Design review of the part built by this model. Coordinates are the model's own, in mm. Face numbers are marked on the shaded views. A direction names the side the tool comes from. Give positions to 0.01 mm unless a question says otherwise; leave off trailing zeros. Write each loop counter-clockwise with the first axis right and the second up, starting at its lowest first coordinate (ties: lowest second). Pieces come first, ordered by that corner, then holes. Notation, with made-up numbers: (77.5, 20.5) -> (124.5, 20.5) arc R27 cw to (124.5, 37.5) -> close; hole circle Ø2 at (37.25, -30.75). An arc over 180 degrees is marked (long way). Return JSON: item names as keys, results as strings. Group by question number.
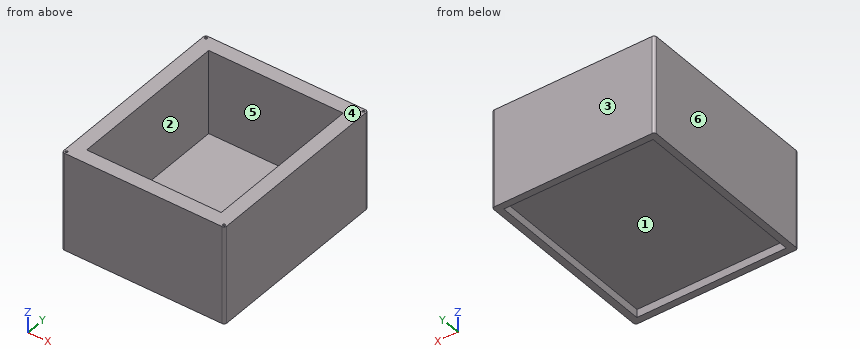
from build123d import *

# Parameters (mm, degrees)
F0_W     = 61.468
F0_H     = 71.628
F0_W_2   = 50.8
F0_H_2   = 60.96
F1_DEPTH = 18.542
F2_W     = 50.8
F2_H     = 60.96
F3_DEPTH = 5.334
F4_R     = 0.9906
F5_T     = -2.54
F6_R     = 0.4445
F7_DEPTH = 3.3782


with BuildPart() as f1:
    # F0 (on Top) → F1 (new body, symmetric)
    with BuildSketch(Plane.XY):
        Rectangle(F0_W, F0_H)
        Rectangle(F0_W_2, F0_H_2, mode=Mode.SUBTRACT)
    extrude(amount=F1_DEPTH, both=True)

    # F2 (on face) → F3 (join)
    with BuildSketch(Plane(origin=(0, 0, -18.542), x_dir=(1, 0, 0), z_dir=(0, 0, -1))):
        Rectangle(F2_W, F2_H)
    extrude(amount=-F3_DEPTH)

    # F4
    f4_edges = [f1.edges().sort_by_distance(p)[0] for p in [
        (-30.734, 35.814, 0),
        (30.734, 35.814, 0),
        (30.734, -35.814, 0),
        (-30.734, -35.814, 0),
    ]]
    fillet(f4_edges, radius=F4_R)

    # F5
    f5_openings = [f1.faces().sort_by_distance(p)[0] for p in [
        (0, 0, -18.542),
    ]]
    offset(amount=F5_T, openings=f5_openings, kind=Kind.INTERSECTION)

    # F6 (on face) → F7 (cut)
    with BuildSketch(Plane.XY.offset(18.542)):
        with Locations((-29.7434, 34.8234)):
            Circle(F6_R)
        with Locations((29.7434, 34.8234)):
            Circle(F6_R)
        with Locations((29.7434, -34.8234)):
            Circle(F6_R)
        with Locations((-29.7434, -34.8234)):
            Circle(F6_R)
    extrude(amount=-F7_DEPTH, mode=Mode.SUBTRACT)


solid = f1.part
Q1. Mouldability with a two-part tool opening along X and no side actions: class the marked faces 4, 5 and 6 as +X half, -X half, draft (parallel to the pull), parting line (faces both ways), or undercut.
Q2. Take a section at A-A, the plane z = 0. Give the boundary of the cut face in (x, y), plus the area to 3 significant figures.
Q3. Insertion check: pin 1 (12 mm diameter, centred on x = 15, y = -25.5, fed in from -Z); pin 2 (6 mm diameter, centred on x = -1, y = 16.5, fed in from +Z). Each pin has a flat end and moves straight along its axis. Give the tip position at first contact, or say it passes through.
Q4. Take a section at C-C, the plane y = 15. Give the boundary of the cut face in (x, z).
Q5. Tool access review of the marked faces 1, 2 and 3: name each direction out of +Z, -Z, +X, -X, +Y, -Y from which nothing blocks a thin tool from reaching the whole face with its end or side.
Q6. Take a section at B-B, the plane x = 19.5. Give the boundary of the cut face in (y, z).
Q7. For L1, parallel to X at y = -28, z = 5.5; L2, parallel to Y at x = 26, z = -4; L3, parallel to Y at x = 19, z = 15, list the stretches that pass through material, from the lowest coordinate up. Write a range as from..to.
Final values:
{
 "1": {"face 4": "draft", "face 5": "undercut", "face 6": "-X half"},
 "2": {"outline": "(-30.73, -34.82) arc R0.99 ccw to (-29.74, -35.81) -> (29.74, -35.81) arc R0.99 ccw to (30.73, -34.82) -> (30.73, 34.82) arc R0.99 ccw to (29.74, 35.81) -> (-29.74, 35.81) arc R0.99 ccw to (-30.73, 34.82) -> close; (-27.94, -33.02) -> (27.94, -33.02) -> (27.94, 33.02) -> (-27.94, 33.02) -> close; hole (-28.19, -33.27) -> (28.19, -33.27) -> (28.19, 33.27) -> (-28.19, 33.27) -> close; hole (-25.4, -30.48) -> (25.4, -30.48) -> (25.4, 30.48) -> (-25.4, 30.48) -> close", "area": "1,240 mm²"},
 "3": {"pin 1": "stops at z = -15.75", "pin 2": "stops at z = -13.21"},
 "4": {"outline": "(-30.73, -18.54) -> (-28.19, -18.54) -> (-28.19, 16) -> (-27.94, 16) -> (-27.94, -15.75) -> (27.94, -15.75) -> (27.94, 16) -> (28.19, 16) -> (28.19, -18.54) -> (30.73, -18.54) -> (30.73, 18.54) -> (25.4, 18.54) -> (25.4, -13.21) -> (-25.4, -13.21) -> (-25.4, 18.54) -> (-30.73, 18.54) -> close"},
 "5": {"face 1": "-Z", "face 2": "+Z", "face 3": "+Z, -Z, +X, -X, +Y"},
 "6": {"outline": "(-35.81, -18.54) -> (-33.27, -18.54) -> (-33.27, 16) -> (-33.02, 16) -> (-33.02, -15.75) -> (33.02, -15.75) -> (33.02, 16) -> (33.27, 16) -> (33.27, -18.54) -> (35.81, -18.54) -> (35.81, 18.54) -> (30.48, 18.54) -> (30.48, -13.21) -> (-30.48, -13.21) -> (-30.48, 18.54) -> (-35.81, 18.54) -> close"},
 "7": {"L1": "x = -30.73..-28.19, -27.94..-25.4, 25.4..27.94, 28.19..30.73", "L2": "y = -35.81..-33.27, -33.02..33.02, 33.27..35.81", "L3": "y = -35.81..-33.27, -33.02..-30.48, 30.48..33.02, 33.27..35.81"}
}
